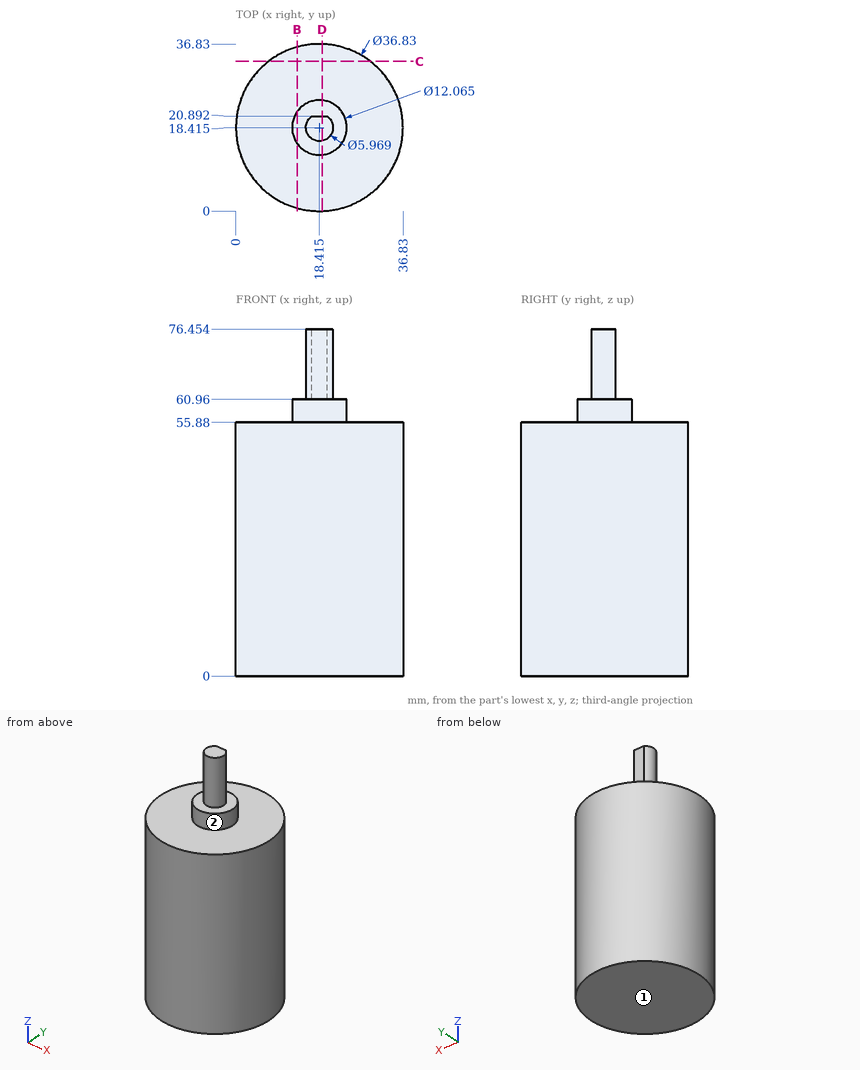
Can you work these out from the drawing? Everything is in mm from the part's minimum corner. A direction names the side the tool comes from. Coordinates: 2 decimals unless noted, no trailing zeros. Loops run counter-clockwise (first coordinate to the right, second up) from the corner with the lowest first, then second, coordinate; pieces in that order, holes last. Notation, with made-up numbers: (8.25, 7.25) - (42.25, 7.25) arc R25 cw to (42.25, 25.25) - close; hole circle Ø6 at (-8.5, 36). An arc over 180 degrees is marked (long way). Put each result on its own line as item: value. Start each with the question number.
Item 1: For pin 1 (12 mm diameter, centred on y = 7.5, z = 22, fed in from -X); pin 2 (12 mm diameter, centred on x = 16, z = 11.5, fed in from +Y); pin 3 (2 mm diameter, centred on x = 10, z = 35.5, fed in from +Y), each with a flat end and sliding along its axis, tell me the tip position at first contact or that it passes through.
Item 2: Suppose I cut it at C-C (y = 33). Please give me the cut outline in (x, z).
Item 3: Suppose I cut it at D-D (x = 19). Please give me the cut outline in (y, z) (1 decimal).
Item 4: Which directions (+Z, -Z, +X, -X, +Y, -Y) give clear straight access to the entire face, cutting with the end or side of a thin tool? Please do the marked faces 1 and 2.
Item 5: If I drill on line 1 along Z through (x, y) = (5.5, 19); line 2 along Z through (x, y) = (14, 16); line 3 along X through (y, z) = (24, 15.5), over which ranges is the centre line in solid material (lowest first)?
Item 6: Suppose I cut it at B-B (x = 13.5). Please give me the cut outline in (y, z).
Here are the results:
1. pin 1: x = 0.67
1. pin 2: y = 36.83
1. pin 3: y = 35.27
2. outline: (7.17, 0) - (29.66, 0) - (29.66, 55.88) - (7.17, 55.88) - close
3. outline: (0, 0) - (36.8, 0) - (36.8, 55.9) - (24.4, 55.9) - (24.4, 61) - (20.9, 61) - (20.9, 76.5) - (15.5, 76.5) - (15.5, 61) - (12.4, 61) - (12.4, 55.9) - (0, 55.9) - close
4. face 1: -Z, +X, -X, +Y, -Y
4. face 2: +Z
5. line 1: 0 to 55.88
5. line 2: 0 to 60.96
5. line 3: 0.87 to 35.96
6. outline: (0.67, 0) - (36.16, 0) - (36.16, 55.88) - (21.91, 55.88) - (21.91, 60.96) - (14.92, 60.96) - (14.92, 55.88) - (0.67, 55.88) - close
